from build123d import *

# Parameters (mm, degrees)
SKETCH2_R           = 2.35
BOSS_EXTRUDE1_DEPTH = 1
SKETCH3_R           = 4
BOSS_EXTRUDE2_DEPTH = 2
SKETCH4_R           = 2.675
CUT_EXTRUDE1_DEPTH  = 1.8
CUT_EXTRUDE1_DRAFT  = -45
SKETCH5_R           = 1.5
CUT_EXTRUDE2_DEPTH  = 1.8
CHAMFER1_SIZE       = 0.5


with BuildPart() as part:
    # Sketch2 → Boss-Extrude1 (new body)
    with BuildSketch(Plane(origin=(0, 0, 0), x_dir=(1, 0, 0), z_dir=(0, 1, 0))):
        with Locations(Location((0, 0, 0), (0, 0, 270))):
            Circle(SKETCH2_R)
    extrude(amount=BOSS_EXTRUDE1_DEPTH)

    # Sketch3 → Boss-Extrude2 (add)
    with BuildSketch(Plane.XZ):
        with Locations(Location((0, 0, 0), (0, 0, 270))):
            Circle(SKETCH3_R)
    extrude(amount=BOSS_EXTRUDE2_DEPTH)


with BuildPart() as cut_extrude1_tool:
    # Sketch4 → Cut-Extrude1 (with draft: the straight prism first)
    with BuildSketch(Plane.XZ.offset(2)):
        Circle(SKETCH4_R)
    extrude(amount=-CUT_EXTRUDE1_DEPTH)
    # Cut-Extrude1: the draft: its side faces are tilted about the plane it starts from
    cut_extrude1_sides = [cut_extrude1_tool.faces().sort_by_distance(p)[0] for p in [
        (-2.675, -1.1, 0),
    ]]
    draft(cut_extrude1_sides, Plane.XZ.offset(2), CUT_EXTRUDE1_DRAFT)


with BuildPart() as part_1:
    add(part.part)

    # Cut-Extrude1: cut by cut_extrude1_tool
    add(cut_extrude1_tool.part, mode=Mode.SUBTRACT)

    # Sketch5 → Cut-Extrude2 (cut)
    with BuildSketch(Plane(origin=(0, 1, 0), x_dir=(1, 0, 0), z_dir=(0, 1, 0))):
        with Locations(Location((0, 0, 0), (0, 0, 270))):
            Circle(SKETCH5_R)
    extrude(amount=-CUT_EXTRUDE2_DEPTH, mode=Mode.SUBTRACT)

    # Chamfer1
    chamfer1_edges = [part_1.edges().sort_by_distance(p)[0] for p in [
        (0, -2, 4),
    ]]
    chamfer(chamfer1_edges, length=CHAMFER1_SIZE)


solid = part_1.part
Check sheet for the modelled part. Datum: model origin and axes. Units: mm. A direction names the side the tool comes from. Give positions to 0.01 mm unless a question says otherwise; leave off trailing zeros. Order: outer loops, then holes, each group sorted by start corner. A loop starts at its lowest first (then second) coordinate and runs counter-clockwise, first axis right, second up. Notation, with made-up numbers: (78.5, -12) - (104.5, -12) arc R28 cw to (104.5, 15) - close; hole circle Ø3 at (25, 54.25). An arc over 180 degrees is marked (long way). Answer as CSV lines item,"result".
1. Go/stop test with flat-tipped pins: P1, Ø2.5, axis at x = 0, z = 0, coming from the +Y side; P2, Ø1.5, axis at y = -1, z = -3, coming from the +X side. Record where each tip stops, or that it passes through.
Result sheet:
P1,"through"
P2,"x = 3.31"
2. Scan lines: probe 1 along X at (y, z) = (0.6, 0); probe 2 along X at (y, z) = (-0.2, 0); probe 3 along Y at (x, z) = (3, 0). Record each from-to range of solid material in increasing order. Write a range as from..to.
Result sheet:
probe 1,"-2.35..-1.5, 1.5..2.35"
probe 2,"-4..-1.5, 1.5..4"
probe 3,"-2..0"
3. Section check C-C (y = 0.25). Record the boundary of the cut face in (x, z), then the cut area to 3 significant figures.
Result sheet:
outline,"circle Ø4.7 at (0, 0); hole circle Ø3 at (0, 0)"
area,"10.3 mm²"
4. Tool access check on faces 1 (the face through (-2, 0, -2)), 2 (the face through (-3.905, -0.74, 0.867)). Record the directions out of +Z, -Z, +X, -X, +Y, -Y that give a thin tool (end or side, any length) a straight path to the whole face; none if there is none.
Result sheet:
face 1,"+Y"
face 2,"+Y, -Y"
5. Section check D-D (y = -0.9). Record the boundary of the cut face in (x, z) (3 decimals).
Result sheet:
outline,"circle Ø8 at (0, 0); hole circle Ø3.15 at (0, 0)"
6. Mould release check, pull along X, two halves, no side actions. Record for faces 3 (the face through (0.71, 0.49, 2.24)), 4 (the face through (0.45, 0.11, 1.43)), 5 (the face through (-3, -2, 1)): released by +X, released by -X, zero draft, split by the parting line, or undercut.
Result sheet:
face 3,"split by the parting line"
face 4,"undercut"
face 5,"zero draft"
7. Section check B-B (z = 0). Record the boundary of the cut face in (x, y) (3 decimals).
Result sheet:
outline,"(-4, -1.5) - (-3.5, -2) - (-2.675, -2) - (-1.475, -0.8) - (-1.5, -0.8) - (-1.5, 1) - (-2.35, 1) - (-2.35, 0) - (-4, 0) - close; (1.475, -0.8) - (2.675, -2) - (3.5, -2) - (4, -1.5) - (4, 0) - (2.35, 0) - (2.35, 1) - (1.5, 1) - (1.5, -0.8) - close"
8. Section check A-A (x = 0). Record the boundary of the cut face in (y, z) (3 decimals), then the cut area to 3 significant figures.
Result sheet:
outline,"(-2, -3.5) - (-1.5, -4) - (0, -4) - (0, -2.35) - (1, -2.35) - (1, -1.5) - (-0.8, -1.5) - (-0.8, -1.475) - (-2, -2.675) - close; (-2, 2.675) - (-0.8, 1.475) - (-0.8, 1.5) - (1, 1.5) - (1, 2.35) - (0, 2.35) - (0, 4) - (-1.5, 4) - (-2, 3.5) - close"
area,"10.1 mm²"
